The listing builds one solid part. Answer for the finished solid, in the listing's coordinates (mm). A direction names the side the tool comes from. Coordinates: 2 decimals unless noted, no trailing zeros. Loops run counter-clockwise (first coordinate to the right, second up) from the corner with the lowest first, then second, coordinate; pieces in that order, holes last. Notation, with made-up numbers: (-24.75, 50) - (11.25, 50) arc R21 ccw to (11.25, 57) - close; hole circle Ø6 at (46.25, 38). An arc over 180 degrees is marked (long way). Return JSON: item names as keys, results as strings. Group by question number.
1. Find the intervals of material crossed by line 1 along Z through (x, y) = (0, -3) (3 decimals); line 2 along Z through (x, y) = (0, -19.25) (3 decimals); line 3 along Y through (x, z) = (6.5, 27), in increasing order.
2. Each of these flat-tipped pins is pushed along its axis until it touches: P1, Ø3, axis at y = -20.5, z = -2.5, coming from the +X side; P2, Ø8, axis at y = -3.5, z = -11.5, coming from the +X side; P3, Ø12, axis at x = -5.5, y = -17.5, coming from the -Z side. Where does it stop, or does it pass through?
3. Section C-C (y = -7.5) is taken. Write down the section's boundary in (x, z) (3 decimals).
4. Which of the six approach directions +Z, -Z, +X, -X, +Y, -Y give full straight-line access (tool end or side, diameter ignored) to faces 1 (the face through (14.274, -12.431, -0.628)), 2 (the face through (-3.441, -20.704, -15.497)), 3 (the face through (-3.441, -4.383, -15.497))?
5. The mould has two halves that part along Z. Classify faces 4 (the face through (-11.83, -15.875, 8.31)), 5 (the face through (2, -6.35, -26)), 6 (the face through (-30.235, -1.565, -23.183)): pulls with the +Z half, pulls with the -Z half, needs draft (parallel to the pull), parting line crosses it, or undercut.
```python
from build123d import *

# Parameters (mm, degrees)
F0_R     = 38.1
F1_DEPTH = 6.35
F2_R     = 25.4
F3_DEPTH = 19.05
F5_D     = 28.575
F6_R     = 15.875
F7_DEPTH = 9.525
F8_R     = 3.175
F4_R     = 15.875
F9_DEPTH = 8.89


with BuildPart() as f1:
    # F0 (on Front) → F1 (new body)
    with BuildSketch(Plane.XZ):
        Circle(F0_R)
    extrude(amount=F1_DEPTH)

    # F2 (on face) → F3 (join)
    with BuildSketch(Plane.XZ.offset(6.35)):
        Circle(F2_R)
    extrude(amount=F3_DEPTH)

    # F5 (through all)
    with Locations(Plane(origin=(0, 0, 0), x_dir=(1, 0, 0), z_dir=(0, 1, 0))):
        with Locations((0, 0)):
            Hole(F5_D / 2)

    # F6 (on face) → F7 (cut)
    with BuildSketch(Plane.XZ.offset(25.4)):
        Circle(F6_R)
    extrude(amount=-F7_DEPTH, mode=Mode.SUBTRACT)

    # F8
    f8_edges = [f1.edges().sort_by_distance(p)[0] for p in [
        (-38.1, -6.35, 0),
    ]]
    fillet(f8_edges, radius=F8_R)

    # F4 (on Front) → F9 (cut)
    with BuildSketch(Plane.XZ):
        Circle(F4_R)
    extrude(amount=F9_DEPTH, mode=Mode.SUBTRACT)


solid = f1.part
```
The answers:
{
 "1": {"line 1": "z = -38.1 to -15.875, 15.875 to 38.1", "line 2": "z = -25.4 to -15.875, 15.875 to 25.4", "line 3": "y = -6.35 to 0"},
 "2": {"P1": "stops at x = 25.38", "P2": "stops at x = 37.35", "P3": "stops at z = -25.4"},
 "3": {"outline": "circle Ø50.8 at (0, 0); hole circle Ø31.75 at (0, 0)"},
 "4": {"face 1": "+Y, -Y", "face 2": "-Y", "face 3": "+Y"},
 "5": {"face 4": "undercut", "face 5": "needs draft", "face 6": "parting line crosses it"}
}
